The listing builds one solid part. Answer for the finished solid, in the listing's coordinates (mm). Face numbers are marked on the shaded views. A direction names the side the tool comes from. Give positions to 0.01 mm unless a question says otherwise; leave off trailing zeros. Write each loop counter-clockwise with the first axis right and the second up, starting at its lowest first coordinate (ties: lowest second). Pieces come first, ordered by that corner, then holes. Notation, with made-up numbers: (3, 60) - (42, 60) arc R9 cw to (42, 72) - close; hole circle Ø7 at (44.5, 30.5). An arc over 180 degrees is marked (long way). Return JSON: item names as keys, results as strings.
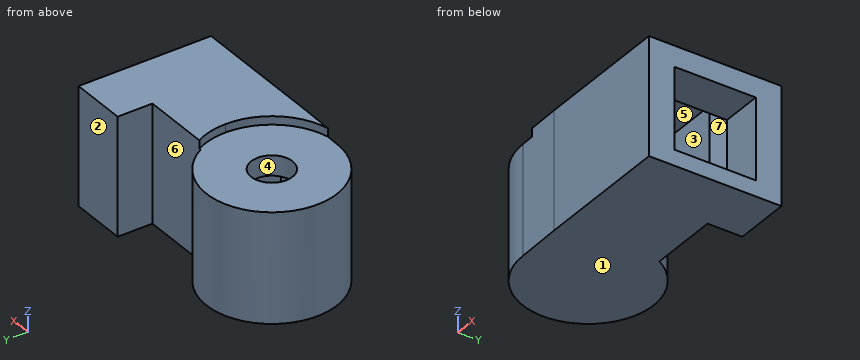
from build123d import *

# Parameters (mm, degrees)
F1_DEPTH  = 71
F2_W      = 49
F2_H      = 49
F3_DEPTH  = 25
F5_W      = 46
F5_H      = 55
F6_DEPTH  = 60
F8_R      = 34.5
F9_DEPTH  = 49
F10_R     = 12.5
F11_DEPTH = 25
F12_R     = 12.5
F13_DEPTH = 5


with BuildPart() as f1:
    # F0 (on Top) → F1 (new body)
    with BuildSketch(Plane.XY):
        with BuildLine():
            ThreePointArc((-35.5, 0.5), (-7.569282, 12.069282), (4, 40))
            ThreePointArc((4, 40), (2.763184, 49.807077), (-0.869811, 59))
            ThreePointArc((-0.869811, 59), (-69.490808, 60.121506), (-35.5, 0.5))
        make_face()
        with BuildLine():
            ThreePointArc((-0.869811, 59), (2.763184, 49.807077), (4, 40))
            ThreePointArc((4, 40), (-7.569282, 12.069282), (-35.5, 0.5))
            Line((-35.5, 0.5), (-7.508424, 0))
            Line((-7.508424, 0), (75, 0))
            Line((75, 0), (75, 80))
            Line((75, 80), (41, 80))
            Line((41, 80), (41, 59))
            Line((41, 59), (-0.869811, 59))
        make_face()
    extrude(amount=F1_DEPTH)

    # F2 (on face) → F3 (cut)
    with BuildSketch(Plane.YZ.offset(75)):
        with Locations((40, 34)):
            Rectangle(F2_W, F2_H)
    extrude(amount=-F3_DEPTH, mode=Mode.SUBTRACT)

    # F5 (on offset) → F6 (cut)
    with BuildSketch(Plane.YZ.offset(50)):
        with Locations((31, 35.5)):
            Rectangle(F5_W, F5_H)
    extrude(amount=-F6_DEPTH, mode=Mode.SUBTRACT)

    # F8 (on offset) → F9 (cut)
    with BuildSketch(Plane.XY.offset(5)):
        with Locations((-35.5, 40)):
            Circle(F8_R)
    extrude(amount=F9_DEPTH, mode=Mode.SUBTRACT)

    # F10 (on face) → F11 (cut)
    with BuildSketch(Plane.XY.offset(71)):
        with Locations((-35.5, 40)):
            Circle(F10_R)
    extrude(amount=-F11_DEPTH, mode=Mode.SUBTRACT)

    # F12 (on face) → F13 (cut)
    with BuildSketch(Plane.XY.offset(71)):
        with BuildLine():
            ThreePointArc((-27.234726, 0.352361), (-4.075538, 14.450965), (5, 40))
            ThreePointArc((5, 40), (3.798839, 49.790366), (0.266605, 59))
            Line((0.266605, 59), (-0.869811, 59))
            ThreePointArc((-0.869811, 59), (-69.490808, 60.121506), (-35.5, 0.5))
            Line((-35.5, 0.5), (-27.234726, 0.352361))
        make_face()
        with Locations((-35.5, 40)):
            Circle(F12_R, mode=Mode.SUBTRACT)
        with BuildLine():
            Line((-0.869811, 59), (0.266605, 59))
            ThreePointArc((0.266605, 59), (-72.168624, 57.194826), (-27.234726, 0.352361))
            Line((-27.234726, 0.352361), (-35.5, 0.5))
            ThreePointArc((-35.5, 0.5), (-69.490808, 60.121506), (-0.869811, 59))
        make_face()
    extrude(amount=-F13_DEPTH, mode=Mode.SUBTRACT)


solid = f1.part
Item 1: Consider L1, parallel to Z at x = 34, y = 22; L2, parallel to Y at x = -35.5, z = 37.5; L3, parallel to Z at x = -10, y = 61. Determine where each line is inside the solid, lowest interval first.
Answer below:
{"L1": "z = 0 to 8, 63 to 71", "L2": "y = 0.5 to 5.5, 74.5 to 79.5", "L3": "z = 0 to 5, 54 to 66"}
Item 2: A cutting plane is placed at B-B on y = 62.5. Determine the outline of the cut face in (x, z).
Answer below:
{"outline": "(-67.97, 0) - (-3.03, 0) - (-3.03, 66) - (-67.97, 66) - close; (41, 0) - (75, 0) - (75, 9.5) - (50, 9.5) - (50, 58.5) - (75, 58.5) - (75, 71) - (41, 71) - close; hole (-61.65, 5) - (-9.35, 5) - (-9.35, 54) - (-61.65, 54) - close"}
Item 3: A cutting plane is placed at A-A on x = 62.5. Determine the outline of the cut face in (y, z), then the cut area to 3 significant figures.
Answer below:
{"outline": "(0, 0) - (80, 0) - (80, 71) - (0, 71) - close; hole (15.5, 9.5) - (64.5, 9.5) - (64.5, 58.5) - (15.5, 58.5) - close", "area": "3,280 mm²"}
Item 4: A cutting plane is placed at D-D on z = 52. Determine the outline of the cut face in (x, y).
Answer below:
{"outline": "(-35.5, 0.5) - (-7.51, 0) - (75, 0) - (75, 15.5) - (50, 15.5) - (50, 8) - (-10, 8) - (-10, 16.76) arc R34.5 cw (long way) to (-3.97, 54) - (50, 54) - (50, 64.5) - (75, 64.5) - (75, 80) - (41, 80) - (41, 59) - (-0.87, 59) arc R39.5 ccw (long way) to start"}
Item 5: For the marked faces 4, 5, 6 and 7, determine the directions among +Z, -Z, +X, -X, +Y, -Y from which every point of the face is accessible in a straight line to the end or side of a thin tool.
Answer below:
{"face 4": "+Z", "face 5": "none", "face 6": "+Z, -Z, +Y", "face 7": "+X"}
Item 6: Flat-ended cylindrical pins translate along their axes: P1, Ø8, axis at x = -12.5, y = 12.5, coming from the +Z side; P2, Ø2, axis at y = 58.5, z = 60, coming from the -X side; P3, Ø1, axis at y = 45, z = 48.5, coming from the +X side. Find the tip coordinate at first contact, or state that the pin passes through.
Answer below:
{"P1": "stops at z = 66", "P2": "stops at x = -70.91", "P3": "stops at x = -69.56"}
Item 7: A cutting plane is placed at C-C on y = 42. Determine the outline of the cut face in (x, z), then the cut area to 3 significant figures.
Answer below:
{"outline": "(-74.95, 0) - (75, 0) - (75, 9.5) - (50, 9.5) - (50, 8) - (-1.06, 8) - (-1.06, 5) - (-69.94, 5) - (-69.94, 54) - (-47.84, 54) - (-47.84, 66) - (-74.95, 66) - close; (-23.16, 54) - (-10, 54) - (-10, 63) - (50, 63) - (50, 58.5) - (75, 58.5) - (75, 71) - (4.95, 71) - (4.95, 66) - (-23.16, 66) - close", "area": "2,460 mm²"}
Item 8: The mould has two halves that part along Y. Classify the marked faces 1, 2 and 3: +Y half, -Y half, draft (parallel to the pull), parting line (faces both ways), or undercut.
Answer below:
{"face 1": "draft", "face 2": "+Y half", "face 3": "undercut"}
